The model under review builds one solid part; all positions refer to its coordinate system, in mm. Face numbers are marked on the shaded views. Round coordinates to 2 decimals unless told otherwise and drop trailing zeros. Loops run counter-clockwise (first coordinate to the right, second up) from the corner with the lowest first, then second, coordinate; pieces in that order, holes last. Notation, with made-up numbers: M -16,51 L -8,51 A24 ccw -8,72 Z; hole C 81,42.5 d7. An arc over 180 degrees is marked long. Return JSON: item names as keys, results as strings. Group by question number.
Q1. Consider section A-A (y = 0). State the section outline as (x, z) points.
Q2. Clearance check with flat-ended pins moving along their axes: pin 1 Ø2 at (y, z) = (-1, 13.5) entering from +X; pin 2 Ø2 at (y, z) = (-5, 7.5) entering from +X; pin 3 Ø1 at (y, z) = (3.5, 22.5) entering from -X; pin 4 Ø8 at (x, z) = (5, 14.5) entering from -Y. State where each tip first meets the part, or that it passes through.
Q3. Consider section D-D (x = -3.5). State the section outline as (y, z) points, and give its area (3 significant figures).
Q4. Consider section C-C (z = 6.5). State the section outline as (x, y) points, and give its area (3 significant figures).
Q5. Consider section B-B (x = 0.75). State the section outline as (y, z) points.
Q6. Draft analysis for pull direction Y (two halves, no side actions). For the marked faces 1, 2 and 3, state which applies: pulls with the +Y half, pulls with the -Y half, needs draft (parallel to the pull), parting line crosses it, or undercut.
Q7. To check wall thickness, follow line 1 along X through (y, z) = (0, 7.75); line 2 along X through (y, z) = (0, 20.75); line 3 along Z through (x, y) = (0, 7). State the ranges of each line that lie inside material, in increasing order.
from build123d import *

# Parameters (mm, degrees)
CYLINDER005_R     = 10.2
CYLINDER005_DEPTH = 4
CYLINDER006_R     = 14
CYLINDER006_DEPTH = 4
BOX_W             = 30
BOX_H             = 30
BOX_DEPTH         = 36
CYLINDER004_R     = 4.5
CYLINDER004_DEPTH = 100
CYLINDER_R        = 7.55
CYLINDER_DEPTH    = 45
CYLINDER001_R     = 10.2
CYLINDER001_DEPTH = 70
CYLINDER002_R     = 13
CYLINDER002_DEPTH = 4
CYLINDER003_R     = 13
CYLINDER003_DEPTH = 4


with BuildPart() as cilindro001:
    # Cylinder005 → Cylinder005 (new body)
    with BuildSketch(Plane.XY):
        Circle(CYLINDER005_R)
    extrude(amount=CYLINDER005_DEPTH)


with BuildPart() as cut003:
    # Cylinder006 → Cylinder006 (new body)
    with BuildSketch(Plane.XY):
        Circle(CYLINDER006_R)
    extrude(amount=CYLINDER006_DEPTH)

    # Cut003: cut Cilindro001
    add(cilindro001.part, mode=Mode.SUBTRACT)


with BuildPart() as cubo:
    # Box → Box (new body)
    with BuildSketch(Plane(origin=(-15, -15, 35), x_dir=(1, 0, 0), z_dir=(0, 0, 1))):
        with Locations((15, 15)):
            Rectangle(BOX_W, BOX_H)
    extrude(amount=BOX_DEPTH)


with BuildPart() as cilindro:
    # Cylinder004 → Cylinder004 (new body)
    with BuildSketch(Plane(origin=(2.4, 0, -14), x_dir=(1, 0, 0), z_dir=(0, 0, 1))):
        Circle(CYLINDER004_R)
    extrude(amount=CYLINDER004_DEPTH)


with BuildPart() as rodamiento:
    # Cylinder → Cylinder (new body)
    with BuildSketch(Plane(origin=(2.4, 0, 12.5), x_dir=(1, 0, 0), z_dir=(0, 0, 1))):
        Circle(CYLINDER_R)
    extrude(amount=CYLINDER_DEPTH)


with BuildPart() as pieza_azul:
    # Cylinder001 → Cylinder001 (new body)
    with BuildSketch(Plane.XY):
        Circle(CYLINDER001_R)
    extrude(amount=CYLINDER001_DEPTH)


with BuildPart() as tapa1:
    # Cylinder002 → Cylinder002 (new body)
    with BuildSketch(Plane.XY):
        Circle(CYLINDER002_R)
    extrude(amount=CYLINDER002_DEPTH)


with BuildPart() as cut004:
    # Cylinder003 → Cylinder003 (new body)
    with BuildSketch(Plane.XY.offset(66)):
        Circle(CYLINDER003_R)
    extrude(amount=CYLINDER003_DEPTH)

    # Fusion: union pieza_azul, tapa1
    add(pieza_azul.part)
    add(tapa1.part)

    # Cut: cut rodamiento
    add(rodamiento.part, mode=Mode.SUBTRACT)

    # Cut001: cut Cilindro
    add(cilindro.part, mode=Mode.SUBTRACT)

    # Cut002: cut Cubo
    add(cubo.part, mode=Mode.SUBTRACT)

    # Cut004: cut Cut003
    add(cut003.part, mode=Mode.SUBTRACT)


solid = cut004.part
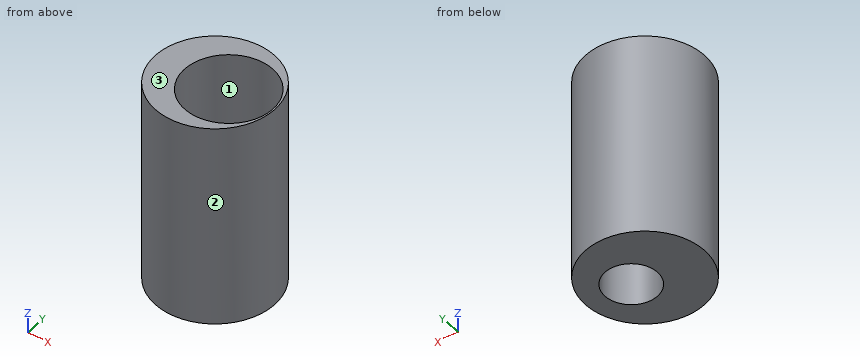
Values:
{
 "1": {"outline": "M -10.2,0 L -2.1,0 L -2.1,12.5 L -5.15,12.5 L -5.15,35 L -10.2,35 Z; M 6.9,0 L 10.2,0 L 10.2,35 L 9.95,35 L 9.95,12.5 L 6.9,12.5 Z"},
 "2": {"pin 1": "stops at x = 10.2", "pin 2": "stops at x = 9.38", "pin 3": "stops at x = -9.75", "pin 4": "stops at y = -10.15"},
 "3": {"outline": "M -9.58,0 L 9.58,0 L 9.58,35 L 4.71,35 L 4.71,12.5 L -4.71,12.5 L -4.71,35 L -9.58,35 Z", "area": "459 mm2"},
 "4": {"outline": "C 0,0 d20.4; hole C 2.4,0 d9", "area": "263 mm2"},
 "5": {"outline": "M -10.17,0 L -4.19,0 L -4.19,12.5 L -7.37,12.5 L -7.37,35 L -10.17,35 Z; M 4.19,0 L 10.17,0 L 10.17,35 L 7.37,35 L 7.37,12.5 L 4.19,12.5 Z"},
 "6": {"face 1": "undercut", "face 2": "parting line crosses it", "face 3": "needs draft"},
 "7": {"line 1": "x = -10.2 to -2.1, 6.9 to 10.2", "line 2": "x = -10.2 to -5.15, 9.95 to 10.2", "line 3": "z = 0 to 12.5"}
}
